Design review of the part built by this model. Coordinates are the model's own, in mm. Face numbers are marked on the shaded views. A direction names the side the tool comes from. Coordinates: 2 decimals unless noted, no trailing zeros. Loops run counter-clockwise (first coordinate to the right, second up) from the corner with the lowest first, then second, coordinate; pieces in that order, holes last. Notation, with made-up numbers: (32.5, -6) -> (55.5, -6) arc R36 cw to (55.5, 28) -> close; hole circle Ø4 at (17, -5.5). An arc over 180 degrees is marked (long way). Answer as a JSON object with one key per item and string values.
```python
from build123d import *

# Parameters (mm, degrees)
F0_R     = 8.95817
F1_DEPTH = 13.716
F2_DEPTH = 76.2
F3_T     = -2.54
F4_R     = 10.281623
F5_DEPTH = 3.175


with BuildPart() as f1:
    # F0 (on Front) → F1 (new body)
    with BuildSketch(Plane.XZ):
        Circle(F0_R)
    extrude(amount=F1_DEPTH)

    # F0 (on Front) → F2 (join)
    with BuildSketch(Plane.XZ):
        Circle(F0_R)
    extrude(amount=F2_DEPTH)

    # F3
    f3_openings = [f1.faces().sort_by_distance(p)[0] for p in [
        (0, -76.2, 0),
    ]]
    offset(amount=F3_T, openings=f3_openings)

    # F4 (on face) → F5 (join)
    with BuildSketch(Plane.XZ.offset(76.2)):
        Circle(F4_R)
    extrude(amount=F5_DEPTH)


solid = f1.part
```
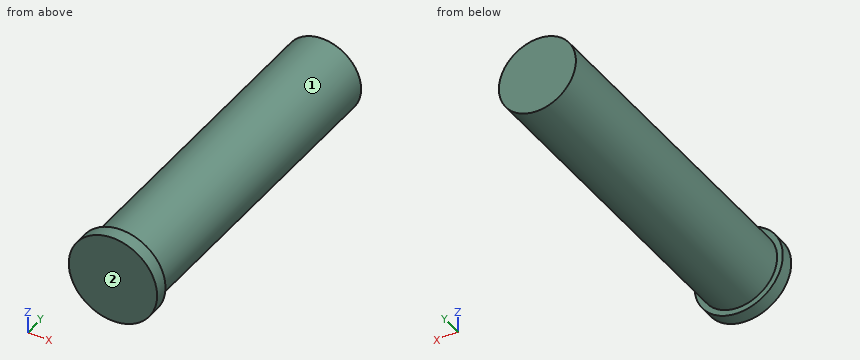
1) Add section A-A, the plane x = 0. Give the boundary of the cut face in (y, z) (3 decimals).
Completed:
{"outline": "(-79.375, -10.282) -> (-76.2, -10.282) -> (-76.2, -8.958) -> (0, -8.958) -> (0, 8.958) -> (-76.2, 8.958) -> (-76.2, 10.282) -> (-79.375, 10.282) -> close; hole (-76.2, -6.418) -> (-2.54, -6.418) -> (-2.54, 6.418) -> (-76.2, 6.418) -> close"}
2) Add section C-C, the plane y = -58.5. Give the boundary of the cut face in (x, z), and give its area (3 significant figures).
Completed:
{"outline": "circle Ø17.92 at (0, 0); hole circle Ø12.84 at (0, 0)", "area": "123 mm²"}
3) Wall thickness on probe 1 along Z at (x, y) = (0, -48); probe 2 along Y at (x, z) = (0.25, -4.5) (3 decimals); probe 3 along X at (y, z) = (-55.5, -2): over which ranges is each line inside the solid? List them lowest first.
Completed:
{"probe 1": "-8.96 to -6.42, 6.42 to 8.96", "probe 2": "-79.375 to -76.2, -2.54 to 0", "probe 3": "-8.73 to -6.1, 6.1 to 8.73"}
4) Add section B-B, the plane z = 0. Give the boundary of the cut face in (x, y) (3 decimals), and give its area (3 significant figures).
Completed:
{"outline": "(-10.282, -79.375) -> (10.282, -79.375) -> (10.282, -76.2) -> (8.958, -76.2) -> (8.958, 0) -> (-8.958, 0) -> (-8.958, -76.2) -> (-10.282, -76.2) -> close; hole (-6.418, -76.2) -> (6.418, -76.2) -> (6.418, -2.54) -> (-6.418, -2.54) -> close", "area": "485 mm²"}
5) Clearance check with flat-ended pins moving along their axes: pin 1 Ø3 at (y, z) = (-64, 2.5) entering from -X; pin 2 Ø1.5 at (x, y) = (1, -12) entering from +Z; pin 3 Ø8 at (y, z) = (-41, -3) entering from +X. State where each tip first meets the part, or that it passes through.
Completed:
{"pin 1": "x = -8.9", "pin 2": "z = 8.95", "pin 3": "x = 8.96"}
6) For the marked faces 1 and 2, list the 3-axis set-ups (+Z, -Z, +X, -X, +Y, -Y) from which the entire face can be reached by the end or side of a thin tool; tool diameter is ignored.
Completed:
{"face 1": "+Y", "face 2": "+Z, -Z, +X, -X, -Y"}
